The model under review builds one solid part; all positions refer to its coordinate system, in mm. Face numbers are marked on the shaded views. A direction names the side the tool comes from. Round coordinates to 2 decimals unless told otherwise and drop trailing zeros. Write each loop counter-clockwise with the first axis right and the second up, starting at its lowest first coordinate (ties: lowest second). Pieces come first, ordered by that corner, then holes. Notation, with made-up numbers: (87, -24) - (123, -24) arc R20 cw to (123, -8) - close; hole circle Ø4 at (81, 86). An arc over 180 degrees is marked (long way). Return JSON: item names as keys, results as strings.
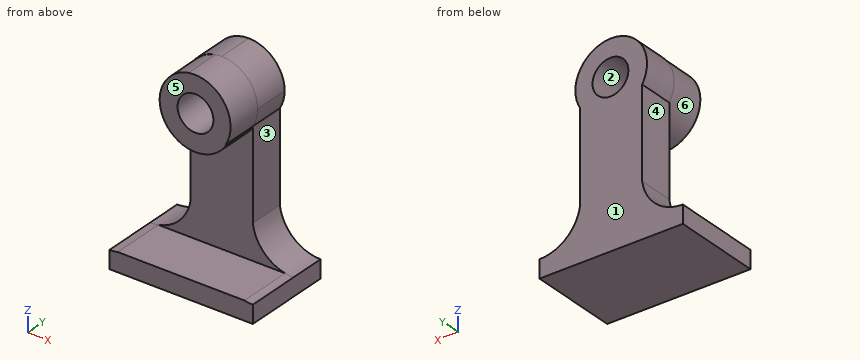
from build123d import *

# Parameters (mm, degrees)
F1_DEPTH = 12.7
F4_DEPTH = 19.05
F6_DEPTH = 12.7
F7_R     = 6.35
F8_DEPTH = 110.49


with BuildPart() as f1:
    # F0 (on Front) → F1 (new body)
    with BuildSketch(Plane.XZ):
        with BuildLine():
            ThreePointArc((27.7772603229, 13.5966521085), (24.0575164439, 22.5769082296), (15.0772603229, 26.2966521085))
            ThreePointArc((15.0772603229, 26.2966521085), (4.0787376948, 19.9466521085), (4.0787376948, 7.2466521085))
            ThreePointArc((4.0787376948, 7.2466521085), (15.0772603229, 0.8966521085), (26.0757829509, 7.2466521085))
            ThreePointArc((26.0757829509, 7.2466521085), (27.3445183167, 10.3096502357), (27.7772603229, 13.5966521085))
        make_face()
        with BuildLine():
            Line((4.0787376948, -24.5033478915), (4.0787376948, -37.2033478915))
            Line((4.0787376948, -37.2033478915), (26.0757829509, -37.2033478915))
            Line((26.0757829509, -37.2033478915), (26.0757829509, -24.5033478915))
            Line((26.0757829509, -24.5033478915), (26.0757829509, 7.2466521085))
            ThreePointArc((26.0757829509, 7.2466521085), (15.0772603229, 0.8966521085), (4.0787376948, 7.2466521085))
            Line((4.0787376948, 7.2466521085), (4.0787376948, -24.5033478915))
        make_face()
        with BuildLine():
            Line((26.0757829509, -24.5033478915), (26.0757829509, -37.2033478915))
            Line((26.0757829509, -37.2033478915), (40.4772603229, -37.2033478915))
            ThreePointArc((40.4772603229, -37.2033478915), (30.876576096, -33.5748251672), (26.0757829509, -24.5033478915))
        make_face()
        with BuildLine():
            ThreePointArc((4.0787376948, -24.5033478915), (-0.7220554503, -33.5748251672), (-10.3227396771, -37.2033478915))
            Line((-10.3227396771, -37.2033478915), (4.0787376948, -37.2033478915))
            Line((4.0787376948, -37.2033478915), (4.0787376948, -24.5033478915))
        make_face()
        Polygon((4.0787376948, -37.2033478915), (-10.3227396771, -37.2033478915), (-10.3227396771, -43.5533478915), (40.4772603229, -43.5533478915), (40.4772603229, -37.2033478915), (26.0757829509, -37.2033478915), align=None)
    extrude(amount=F1_DEPTH)

    # F3 (on face) → F4 (join)
    with BuildSketch(Plane.XZ.offset(12.7)):
        with BuildLine():
            ThreePointArc((40.4772603229, -37.2033478915), (38.989932999, -37.1269472667), (37.5182624684, -36.8985496461))
            Line((37.5182624684, -36.8985496461), (-7.3637418227, -36.8985496461))
            ThreePointArc((-7.3637418227, -36.8985496461), (-8.8354123533, -37.1269472667), (-10.3227396771, -37.2033478915))
            Line((-10.3227396771, -37.2033478915), (-10.3227396771, -43.5533478915))
            Line((-10.3227396771, -43.5533478915), (40.4772603229, -43.5533478915))
            Line((40.4772603229, -43.5533478915), (40.4772603229, -37.2033478915))
        make_face()
    extrude(amount=F4_DEPTH)

    # F5 (on face) → F6 (join)
    with BuildSketch(Plane.XZ.offset(12.7)):
        with BuildLine():
            ThreePointArc((26.0757829509, 7.2466521085), (25.482031486, 20.8788727205), (12.8772183881, 26.1046421743))
            ThreePointArc((12.8772183881, 26.1046421743), (4.8688817883, 6.4640315912), (26.0757829509, 6.8569466568))
            Line((26.0757829509, 6.8569466568), (26.0757829509, 7.2466521085))
        make_face()
    extrude(amount=F6_DEPTH)

    # F7 (on face) → F8 (cut)
    with BuildSketch(Plane.XZ.offset(25.4)):
        with Locations((15.3429014608, 13.6462952942)):
            Circle(F7_R)
    extrude(amount=-F8_DEPTH, mode=Mode.SUBTRACT)


solid = f1.part
(1) Add section C-C (y = -26.5). Write out the cut boundary in (x, z), plus the area to 3 significant figures.
Filled in:
{"outline": "(-10.32, -43.55) - (40.48, -43.55) - (40.48, -37.2) arc R14.52 cw to (37.52, -36.9) - (-7.36, -36.9) arc R14.52 cw to (-10.32, -37.2) - close", "area": "337 mm2"}
(2) Add section B-B (y = -15.5). Write out the cut boundary in (x, z), plus the area to 3 significant figures.
Filled in:
{"outline": "(-10.32, -43.55) - (40.48, -43.55) - (40.48, -37.2) arc R14.52 cw to (37.52, -36.9) - (-7.36, -36.9) arc R14.52 cw to (-10.32, -37.2) - close; (12.88, 26.1) arc R12.7 ccw (long way) to (26.08, 6.86) - (26.08, 7.25) arc R12.7 ccw to start; hole circle Ø12.7 at (15.34, 13.65)", "area": "711 mm2"}
(3) Add section A-A (x = 20). Write out the cut boundary in (y, z).
Filled in:
{"outline": "(-31.75, -43.55) - (0, -43.55) - (0, 9.33) - (-25.4, 9.33) - (-25.4, 1.83) - (-12.7, 1.83) - (-12.7, -36.9) - (-31.75, -36.9) - close; (-25.4, 17.96) - (0, 17.96) - (0, 25.3) - (-25.4, 25.3) - close"}
(4) Clearance check with flat-ended pins moving along their axes: pin 1 Ø4 at (y, z) = (-5, -12) entering from -X; pin 2 Ø12.5 at (x, z) = (11.5, 18) entering from -Y; pin 3 Ø12 at (x, z) = (1, -31) entering from +Y; pin 4 Ø12.5 at (y, z) = (-15, -8) entering from +X. State where each tip first meets the part, or that it passes through.
Filled in:
{"pin 1": "stops at x = 4.08", "pin 2": "stops at y = -25.4", "pin 3": "stops at y = 0", "pin 4": "stops at x = 26.08"}
(5) Add section D-D (z = -19). Write out the cut boundary in (x, y).
Filled in:
{"outline": "(4.08, -12.7) - (26.08, -12.7) - (26.08, 0) - (4.08, 0) - close"}
(6) For the marked faces 4, 5 and 6, list the 3-axis set-ups (+Z, -Z, +X, -X, +Y, -Y) from which the entire face can be reached by the end or side of a thin tool; tool diameter is ignored.
Filled in:
{"face 4": "-X, +Y, -Y", "face 5": "+Z, +X, -X, -Y", "face 6": "-Y"}
(7) Wall thickness on line 1 (Z direction, x = 18, y = -18.5); line 2 (Z direction, x = 13, y = -14.5); line 3 (X direction, y = -8, z = -23): over which ranges is each line inside the solid? List them lowest first.
Filled in:
{"line 1": "z = -43.55 to -36.9, 1.23 to 7.88, 19.41 to 25.96", "line 2": "z = -43.55 to -36.9, 1.16 to 7.74, 19.55 to 26.13", "line 3": "x = 4.08 to 26.08"}
(8) Mouldability with a two-part tool opening along X and no side actions: class the marked faces 1, 2 and 3 as released by +X, released by -X, zero draft, split by the parting line, or undercut.
Filled in:
{"face 1": "zero draft", "face 2": "undercut", "face 3": "released by +X"}
